```python
from build123d import *

# Parameters (mm, degrees)
SKETCH2_W           = 74
SKETCH2_H           = 76
BOSS_EXTRUDE1_DEPTH = 10
BOSS_EXTRUDE2_DEPTH = 10
HOLE1_D             = 10
CUT_EXTRUDE1_START  = -145
CUT_EXTRUDE1_DEPTH  = 10
CUT_EXTRUDE2_DEPTH  = 64


with BuildPart() as part:
    # Sketch1 → Revolve1 (revolve)
    with BuildSketch(Plane.XY, mode=Mode.PRIVATE) as revolve1_sk:
        Polygon((-77.5, 0), (-77.5, 30), (-67.5, 30), (-67.5, 21), (-27.5, 21), (-27.5, 15), (77.5, 15), (77.5, 0), align=None)
    revolve(revolve1_sk.sketch.rotate(Axis((77.5, 0, 0), (-1, 0, 0)), 90), axis=Axis((77.5, 0, 0), (-1, 0, 0)))

    # Sketch2 → Boss-Extrude1 (add)
    with BuildSketch(Plane.ZY.offset(77.5)):
        Rectangle(SKETCH2_W, SKETCH2_H)
    extrude(amount=BOSS_EXTRUDE1_DEPTH)

    # Sketch3 → Boss-Extrude2 (add)
    with BuildSketch(Plane(origin=(0, 0, -37), x_dir=(-1, 0, 0), z_dir=(0, 0, -1))):
        with BuildLine():
            Line((87.5, 38), (137.149569367, 13.445565337))
            ThreePointArc((137.149569367, 13.445565337), (145.5, 0), (137.149569367, -13.445565337))
            Line((137.149569367, -13.445565337), (87.5, -38))
            Line((87.5, -38), (77.5, -38))
            Line((77.5, -38), (77.5, 38))
            Line((77.5, 38), (87.5, 38))
        make_face()
    boss_extrude2 = extrude(amount=-BOSS_EXTRUDE2_DEPTH)

    # Mirror1: Boss-Extrude2 across plane
    add(boss_extrude2.mirror(Plane.XY))

    # Hole1 (through all)
    with Locations(Plane(origin=(0, 0, -37), x_dir=(-1, 0, 0), z_dir=(0, 0, -1))):
        with Locations((130.5, 0)):
            Hole(HOLE1_D / 2)

    # Sketch8 → Cut-Extrude1 (cut)
    with BuildSketch(Plane(origin=(77.5, 0, 0), x_dir=(0, 0, -1), z_dir=(1, 0, 0)).offset(CUT_EXTRUDE1_START)):
        with BuildLine():
            Line((25, 16.583123952), (25, -16.583123952))
            ThreePointArc((25, -16.583123952), (30, 0), (25, 16.583123952))
        make_face()
        with BuildLine():
            Line((-25, 16.583123952), (-25, -16.583123952))
            ThreePointArc((-25, -16.583123952), (-30, 0), (-25, 16.583123952))
        make_face()
    extrude(amount=-CUT_EXTRUDE1_DEPTH, mode=Mode.SUBTRACT)

    # Sketch9 → Cut-Extrude2 (cut)
    with BuildSketch(Plane(origin=(77.5, 0, 0), x_dir=(0, 0, -1), z_dir=(1, 0, 0))):
        with BuildLine():
            Line((7.5, 12.990381057), (7.5, -12.990381057))
            ThreePointArc((7.5, -12.990381057), (15, 0), (7.5, 12.990381057))
        make_face()
    extrude(amount=-CUT_EXTRUDE2_DEPTH, mode=Mode.SUBTRACT)


solid = part.part
```
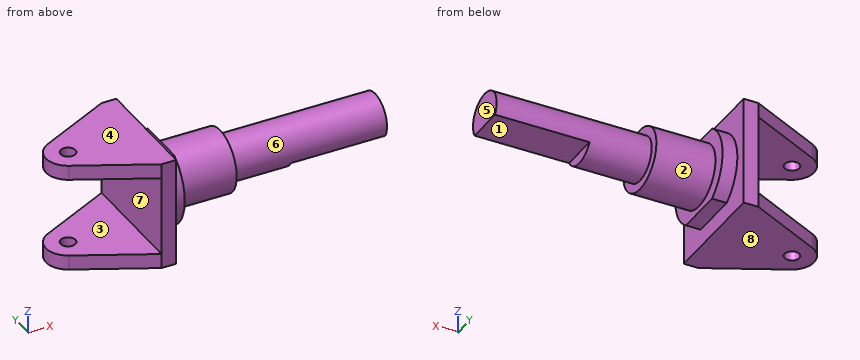
Geometry check sheet. Reference: the model listing, model coordinates, mm. Face numbers are marked on the shaded views. A direction names the side the tool comes from. Give positions to 0.01 mm unless a question says otherwise; leave off trailing zeros. Loops run counter-clockwise (first coordinate to the right, second up) from the corner with the lowest first, then second, coordinate; pieces in that order, holes last. Notation, with made-up numbers: M 10,46 L 14,46 A18 ccw 14,51 Z; hole C -18,25 d1. An arc over 180 degrees is marked long. Write item = value, one per line.
(1) Sectioned sample at C-C, the plane z = 0. Record the cut outline in (x, y), plus the area to 3 significant figures.
Answer below:
outline = M -87.5,-38 L -77.5,-38 L -77.5,-30 L -67.5,-30 L -67.5,-21 L -27.5,-21 L -27.5,-15 L 77.5,-15 L 77.5,15 L -27.5,15 L -27.5,21 L -67.5,21 L -67.5,30 L -77.5,30 L -77.5,38 L -87.5,38 Z
area = 6,190 mm2
(2) Release check for a two-part mould opening along Z. For the marked faces 5, 6, 7 and 8 record: released by +Z, released by -Z, zero draft, split by the parting line, or undercut.
Answer below:
face_5 = zero draft
face_6 = split by the parting line
face_7 = undercut
face_8 = released by -Z
(3) Gauge pin test, flat ends, axial feed: pin 1 Ø6 at (y, z) = (3, -12.5) entering from +X; pin 2 Ø8 at (x, z) = (-61.5, -14) entering from +Y; pin 3 Ø1.5 at (x, z) = (-32, -6) entering from -Y; pin 4 Ø8 at (x, z) = (-112, -22) entering from +Y. Record the tip position at first contact, or that the pin passes through.
Answer below:
pin_1 = 13.5
pin_2 = 18.47
pin_3 = -20.33
pin_4 = through
(4) Tool access check on the marked faces 1, 2, 3 and 4. Record the directions out of +Z, -Z, +X, -X, +Y, -Y that give a thin tool (end or side, any length) a straight path to the whole face; none if there is none.
Answer below:
face_1 = -Z, +X, +Y, -Y
face_2 = +X
face_3 = -X, +Y, -Y
face_4 = +Z, +X, -X, +Y, -Y
(5) Sectioned sample at A-A, the plane y = 0. State how many separate pieces and enclosed holes the cut face has, plus the area to 3 significant figures.
Answer below:
separate_pieces = 3
enclosed_holes = 0
area = 6,550 mm2
(6) Sectioned sample at D-D, the plane y = 11. Record the cut outline in (x, z).
Answer below:
outline = M -140.7,-37 L -77.5,-37 L -77.5,-25 L -67.5,-25 L -67.5,-17.89 L -27.5,-17.89 L -27.5,-10.2 L 13.5,-10.2 L 13.5,-7.5 L 77.5,-7.5 L 77.5,10.2 L -27.5,10.2 L -27.5,17.89 L -67.5,17.89 L -67.5,25 L -77.5,25 L -77.5,37 L -140.7,37 L -140.7,27 L -87.5,27 L -87.5,-27 L -140.7,-27 Z
(7) Sectioned sample at B-B, the plane x = -118. Record the cut outline in (y, z).
Answer below:
outline = M -22.92,-37 L 22.92,-37 L 22.92,-27 L -22.92,-27 Z; M -22.92,27 L 22.92,27 L 22.92,37 L -22.92,37 Z
(8) Material ranges on line 1 (Z direction, x = -101, y = -11); line 2 (Y direction, x = -59, z = -16.5); line 3 (Y direction, x = -130.5, z = -29.75), recorded low to high. Write a range as [from, to].
Answer below:
line_1 = [-37, -27], [27, 37]
line_2 = [-12.99, 12.99]
line_3 = [-16.73, -5], [5, 16.73]
